from build123d import *

# Parameters (mm, degrees)
F0_R     = 14
F0_R_2   = 5.5
F1_DEPTH = 1.5
F0_R_3   = 4
F2_DEPTH = 2.2
F3_DEPTH = 2.2
F4_R     = 4
F5_DEPTH = 3


with BuildPart() as f1:
    # F0 (on Top) → F1 (new body)
    with BuildSketch(Plane.XY):
        with Locations((24.702849, 0.210536)):
            Circle(F0_R)
        with Locations((24.702849, 0.210536)):
            Circle(F0_R_2, mode=Mode.SUBTRACT)
    extrude(amount=F1_DEPTH)

    # F0 (on Top) → F2 (join)
    with BuildSketch(Plane.XY):
        with Locations((24.702849, 0.210536)):
            Circle(F0_R_2)
        with Locations((24.702849, 0.210536)):
            Circle(F0_R_3, mode=Mode.SUBTRACT)
    extrude(amount=F2_DEPTH)

    # F0 (on Top) → F3 (join)
    with BuildSketch(Plane.XY):
        with Locations((24.702849, 0.210536)):
            Circle(F0_R_3)
    extrude(amount=F3_DEPTH)

    # F4 (on face) → F5 (join)
    with BuildSketch(Plane.XY.offset(2.2)):
        with Locations((24.702849, 0.210536)):
            Circle(F4_R)
    extrude(amount=F5_DEPTH)


solid = f1.part
For this review, take the finished solid that the model builds, in its own axes (mm). A direction names the side the tool comes from. Give positions to 0.01 mm unless a question says otherwise; leave off trailing zeros. Loops run counter-clockwise (first coordinate to the right, second up) from the corner with the lowest first, then second, coordinate; pieces in that order, holes last. Notation, with made-up numbers: M 32.25,7 L 84.25,7 A26 cw 84.25,24 Z; hole C 81.5,45 d4. An arc over 180 degrees is marked long. Put each result on its own line as item: value. Start each with the question number.
(1) For pin 1 (1.5 mm diameter, centred on x = 19, z = 0.5, fed in from +Y); pin 2 (2 mm diameter, centred on x = 32, y = -1.5, fed in from -Z); pin 3 (1 mm diameter, centred on y = 2.5, z = 3, fed in from +X); pin 4 (1.5 mm diameter, centred on y = -2.5, z = 4, fed in from -X), all flat-tipped, find the tip position at first contact; note any pin that passes through.
(2) Wall thickness on L1, parallel to Z at x = 20.5, y = 9.75; L2, parallel to Z at x = 27.75, y = -3.25; L3, parallel to X at y = 0, z = 2.8: over which ranges is each line inside the solid? List them lowest first.
(3) Add section D-D, the plane z = 2.9. Write out the cut boundary in (x, y), then the cut area to 3 significant figures.
(4) Add section A-A, the plane x = 29.25. Write out the cut boundary in (y, z), then the cut area to 3 significant figures.
(5) Machinability: for faces 1 (the cylindrical face through (29.78, -1.9, 1.85)), 2 (the cylindrical face through (37.635, -5.152, 0.74)), which of the approach directions +Z, -Z, +X, -X, +Y, -Y give a long, thin tool a straight path to every point of the face, cutting with its end or side? Answer none if there is none.
(6) Add section B-B, the plane y = 3. Write out the cut boundary in (x, z).
(7) Add section C-C, the plane x = 24. Write out the cut boundary in (y, z), then the cut area to 3 significant figures.
Result:
1. pin 1: stops at y = 13.31
1. pin 2: stops at z = 0
1. pin 3: stops at x = 28.28
1. pin 4: stops at x = 21.22
2. L1: z = 0 to 1.5
2. L2: z = 0 to 2.2
2. L3: x = 20.71 to 28.7
3. outline: C 24.7,0.21 d8
3. area: 50.3 mm^2
4. outline: M -13.03,0 L 13.45,0 L 13.45,1.5 L 3.3,1.5 L 3.3,2.2 L -2.88,2.2 L -2.88,1.5 L -13.03,1.5 Z
4. area: 44.1 mm^2
5. face 1: +Z
5. face 2: +Z, -Z
6. outline: M 10.98,0 L 38.42,0 L 38.42,1.5 L 29.44,1.5 L 29.44,2.2 L 27.57,2.2 L 27.57,5.2 L 21.84,5.2 L 21.84,2.2 L 19.96,2.2 L 19.96,1.5 L 10.98,1.5 Z
7. outline: M -13.77,0 L 14.19,0 L 14.19,1.5 L 5.67,1.5 L 5.67,2.2 L 4.15,2.2 L 4.15,5.2 L -3.73,5.2 L -3.73,2.2 L -5.24,2.2 L -5.24,1.5 L -13.77,1.5 Z
7. area: 73.2 mm^2
